```python
from build123d import *

# Parameters (mm, degrees)
SKETCH1_W                                           = 80
SKETCH1_H                                           = 230
BOSS_EXTRUDE1_DEPTH                                 = 6
F_32_0_32_DIAMETER_HOLE1_D                          = 32
FILLET1_R                                           = 30
CBORE_FOR_M3_HEX_SOCKET_HEAD_CAP_SCREW1_D           = 3.4
CBORE_FOR_M3_HEX_SOCKET_HEAD_CAP_SCREW1_CBORE_D     = 6.5
CBORE_FOR_M3_HEX_SOCKET_HEAD_CAP_SCREW1_CBORE_DEPTH = 3.4
SKETCH10_W                                          = 80
SKETCH10_H                                          = 10
CUT_EXTRUDE1_DEPTH                                  = 244.589819163


with BuildPart() as part:
    # Sketch1 → Boss-Extrude1 (new body)
    with BuildSketch(Plane(origin=(0, 0, 0), x_dir=(1, 0, 0), z_dir=(0, 1, 0))):
        with Locations((40, -115)):
            Rectangle(SKETCH1_W, SKETCH1_H)
    extrude(amount=BOSS_EXTRUDE1_DEPTH)

    # Ø32.0 (32) Diameter Hole1 (through all)
    with Locations(Plane(origin=(0, 6, 0), x_dir=(1, 0, 0), z_dir=(0, 1, 0))):
        with Locations((40, -192)):
            Hole(F_32_0_32_DIAMETER_HOLE1_D / 2)

    # Fillet1
    fillet1_edges = [part.edges().sort_by_distance(p)[0] for p in [
        (80, 3, 230),
        (0, 3, 230),
    ]]
    fillet(fillet1_edges, radius=FILLET1_R)

    # CBORE for M3 Hex Socket Head Cap Screw1 (through all)
    with Locations(Plane.XZ):
        with Locations((8, 18), (40, 18), (72, 18), (40, 34), (72, 34), (8, 34)):
            CounterBoreHole(CBORE_FOR_M3_HEX_SOCKET_HEAD_CAP_SCREW1_D / 2, CBORE_FOR_M3_HEX_SOCKET_HEAD_CAP_SCREW1_CBORE_D / 2, CBORE_FOR_M3_HEX_SOCKET_HEAD_CAP_SCREW1_CBORE_DEPTH)

    # Sketch10 → Cut-Extrude1 (cut, through all)
    with BuildSketch(Plane(origin=(0, 6, 0), x_dir=(1, 0, 0), z_dir=(0, 1, 0))):
        with Locations((40, -5)):
            Rectangle(SKETCH10_W, SKETCH10_H)
    extrude(amount=-CUT_EXTRUDE1_DEPTH, mode=Mode.SUBTRACT)


solid = part.part
```
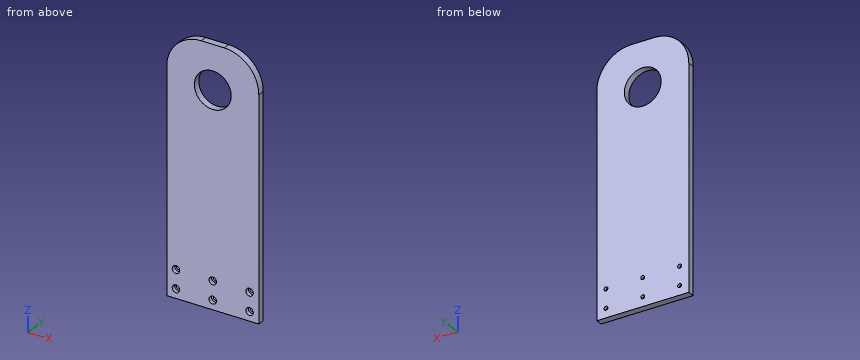
Work out the finished part from the listing and answer in its coordinate system (mm). Give positions to 0.01 mm unless a question says otherwise; leave off trailing zeros. Loops run counter-clockwise (first coordinate to the right, second up) from the corner with the lowest first, then second, coordinate; pieces in that order, holes last. Notation, with made-up numbers: M 19.5,75 L 37.5,75 A23 ccw 37.5,107 Z; hole C 25.5,3.25 d8. An arc over 180 degrees is marked long. One line per item, written item: value. Start each with the question number.
1. This flat-tipped pin is pushed along its axis until it touches: P1, Ø2, axis at x = 41.5, z = 17, coming from the -Y side. Where does it stop, or does it pass through?
2. Find section C-C (x = 33). Give the vertices of the cut face in (y, z), and give its area (3 significant figures).
3. Find the intervals of material crossed by probe 1 along Z at (x, y) = (40, 5); probe 2 along Z at (x, y) = (40, 3.05); probe 3 along Z at (x, y) = (8, 0.85), in increasing order.
4. Find section A-A (y = 4.8). Give the vertices of the cut face in (x, z), and give its area (3 significant figures).
5. Find section B-B (z = 192). Give the vertices of the cut face in (x, y).
Reported:
1. P1: stops at y = 3.4
2. outline: M 0,10 L 6,10 L 6,177.61 L 0,177.61 Z; M 0,206.39 L 6,206.39 L 6,230 L 0,230 Z
2. area: 1,150 mm²
3. probe 1: z = 10 to 16.3, 19.7 to 32.3, 35.7 to 176, 208 to 230
3. probe 2: z = 10 to 14.75, 21.25 to 30.75, 37.25 to 176, 208 to 230
3. probe 3: z = 10 to 14.75, 21.25 to 30.75, 37.25 to 220.4
4. outline: M 0,10 L 80,10 L 80,200 A30 ccw 50,230 L 30,230 A30 ccw 0,200 Z; hole C 8,18 d3.4; hole C 8,34 d3.4; hole C 40,192 d32; hole C 40,18 d3.4; hole C 40,34 d3.4; hole C 72,18 d3.4; hole C 72,34 d3.4
4. area: 16,400 mm²
5. outline: M 0,0 L 24,0 L 24,6 L 0,6 Z; M 56,0 L 80,0 L 80,6 L 56,6 Z
